Geometry check sheet. Reference: the model listing, model coordinates, mm. A direction names the side the tool comes from. Coordinates: 2 decimals unless noted, no trailing zeros. Loops run counter-clockwise (first coordinate to the right, second up) from the corner with the lowest first, then second, coordinate; pieces in that order, holes last. Notation, with made-up numbers: (30.5, -8.75) - (72.5, -8.75) arc R24 ccw to (72.5, 21.25) - close; hole circle Ø11 at (43, 42.5). An arc over 180 degrees is marked (long way). Write item = value, one per line. Start each with the question number.
Autodesk Inventor part; units mm, degrees
ref_plane "YZ Plane" through (0, 0, 0) normal (1, 0, 0) x (0, 1, 0)
ref_plane "XZ Plane" through (0, 0, 0) normal (0, 1, 0) x (-1, 0, 0)
ref_plane "XY Plane" through (0, 0, 0) normal (0, 0, 1) x (1, 0, 0)
sketch "Sketch1" plane through (0, 0, 0) normal (0, 0, 1) x (1, 0, 0)
  line L0 (0, 0) -> (160, 0)
  line L1 (160, 0) -> (118.589, 154.5481)
  line L2 (41.411, 154.5481) -> (0, 0)
  line L3 (41.411, 154.5481) -> (118.589, 154.5481)
  dimension "d0" = 160
  dimension "d1" = 160
  dimension "d2" = 75
  dimension "d8" = 75
extrude "Extrusion1" add sketch "Sketch1" along normal blind 55
sketch "Sketch6" plane through (0, 0, 55) normal (0, 0, 1) x (1, 0, 0)
  line L0 (0, 0) -> (160, 0) construction
  line L1 (160, 0) -> (118.589, 154.5481) construction
  line L2 (118.589, 154.5481) -> (41.411, 154.5481) construction
  line L3 (41.411, 154.5481) -> (0, 0) construction
  line L4 (110.9157, 144.5481) -> (146.9677, 10) construction
  line L5 (146.9677, 10) -> (13.0323, 10) construction
  line L6 (13.0323, 10) -> (49.0843, 144.5481) construction
  line L7 (49.0843, 144.5481) -> (110.9157, 144.5481) construction
  line L8 (85, 144.5481) -> (75, 144.5481) construction
  line L9 (75, 144.5481) -> (75, 10) construction
  line L10 (75, 10) -> (85, 10) construction
  line L11 (85, 10) -> (85, 144.5481) construction
  line L12 (133.5703, 60) -> (26.4297, 60) construction
  line L13 (26.4297, 60) -> (26.4297, 70) construction
  line L14 (26.4297, 70) -> (133.5703, 70) construction
  line L15 (133.5703, 70) -> (133.5703, 60) construction
  line L16 (133.5703, 60) -> (146.9677, 10)
  line L17 (85, 10) -> (146.9677, 10)
  line L18 (0, 0) -> (160, 0) construction
  line L19 (133.5703, 60) -> (85, 60)
  line L20 (85, 60) -> (85, 10)
  line L21 (75, 10) -> (75, 60)
  line L22 (26.4297, 60) -> (75, 60)
  line L23 (26.4297, 60) -> (13.0323, 10)
  line L24 (13.0323, 10) -> (75, 10)
  line L25 (75, 70) -> (75, 144.5481)
  line L26 (75, 144.5481) -> (49.0843, 144.5481)
  line L27 (75, 70) -> (29.1092, 70)
  line L28 (29.1092, 70) -> (49.0843, 144.5481)
  line L29 (85, 144.5481) -> (110.9157, 144.5481)
  line L30 (110.9157, 144.5481) -> (130.8908, 70)
  line L31 (130.8908, 70) -> (85, 70)
  line L32 (85, 70) -> (85, 144.5481)
  point P0 (80, 10)
  dimension "d22" = 10
  dimension "d23" = 10
  dimension "d24" = 10
  dimension "d25" = 50
extrude "Extrusion5" cut sketch "Sketch6" against normal through all
sketch "Sketch7" plane through (0, 0, 0) normal (0, 0, -1) x (-1, 0, 0)
  circle A0 centre (-80, 304.672) radius 315 construction
  line L0 (0, 0) -> (-160, 0)
  arc A1 (-160, 0) -> (0, 0) centre (-80, 304.672) ccw
  dimension "d28" = 630
extrude "Extrusion6" add sketch "Sketch7" against normal blind 55
sketch "Sketch8" plane through (0, 0, 0) normal (0, 0, -1) x (-1, 0, 0)
  circle A0 centre (-80, 4.836) radius 8.25
  line L0 (-15.7117, 20) -> (-144.2883, 20) construction
  line L1 (-13.0323, 10) -> (-15.7117, 20)
  line L2 (-15.7117, 20) -> (-75, 20)
  line L3 (-75, 10) -> (-75, 60)
  line L4 (-75, 20) -> (-75, 10)
  line L5 (-75, 10) -> (-13.0323, 10)
  line L6 (-75, 10) -> (-13.0323, 10)
  line L7 (-26.4297, 60) -> (-13.0323, 10)
  line L8 (-85, 10) -> (-146.9677, 10)
  line L9 (-146.9677, 10) -> (-144.2883, 20)
  line L10 (-133.5703, 60) -> (-146.9677, 10)
  line L11 (-144.2883, 20) -> (-85, 20)
  line L12 (-85, 60) -> (-85, 10)
  line L13 (-85, 20) -> (-85, 10)
  line L14 (-85, 10) -> (-146.9677, 10)
  line L15 (-118.589, 154.5481) -> (-41.411, 154.5481)
  arc A1 (-160, 0) -> (0, 0) centre (-80, 304.672) ccw
  line L16 (0, -10.328) -> (-160, -10.328) construction
  arc A2 (-160, 0) -> (0, 0) centre (-80, 304.672) ccw
  line L17 (-0.263, 4.836) -> (-159.737, 4.836) construction
  point P0 (-80, 154.5481)
  dimension "d31" = 16.5
  dimension "d32" = 20
extrude "Extrusion8" add sketch "Sketch8" against normal blind 55 contours L5 L3 A0 | A0 L3 L2 L1 L5 | L8 L9 L11 L12 A0 | A0 L12 L8
extrude "Extrusion7" cut sketch "Sketch8" against normal through all contours A0 L8 L12 L3 L5 | L5 L3 A0 | A0 L12 L8
sketch "Sketch9" plane through (15.7117, 20, 0) normal (0, 1, 0) x (1, 0, 0)
  line L0 (0, 0) -> (59.2883, 0)
  line L1 (0, -55) -> (0, 0)
  line L2 (59.2883, -55) -> (0, -55)
  line L3 (59.2883, 0) -> (59.2883, -55)
  line L4 (69.2883, 0) -> (128.5765, 0)
  line L5 (69.2883, -55) -> (69.2883, 0)
  line L6 (128.5765, -55) -> (69.2883, -55)
  line L7 (128.5765, 0) -> (128.5765, -55)
  circle A0 centre (29.6441, -27.5) radius 15
  circle A1 centre (98.9324, -27.5) radius 15
  point P0 (-15.7117, 0)
  point P1 (29.6441, 0)
  point P2 (98.9324, 0)
  point P3 (0, -27.5)
  point P4 (69.2883, -27.5)
  dimension "d37" = 30
  dimension "d38" = 30
extrude "Extrusion9" cut sketch "Sketch9" against normal through all contours A0 | A1
properties part number "CA001" material "ABS Plastic"
(1) Sectioned sample at D-D on x = 53. Enter the section's corners in (y, z), plus the area to 3 significant figures.
(2) Scan lines: line 1 (Y direction, x = 60, z = 5); line 2 (Y direction, x = 90.5, z = 8.5); line 3 (Y direction, x = 54, z = 22). Record each from-to range of solid material in increasing order.
(3) Depth check by flat-ended pin: pin 1 (4 mm diameter, centred on y = 95.5, z = 22.5, fed in from +X); pin 2 (8 mm diameter, centred on x = 65.5, z = 26.5, fed in from -Y); pin 3 (10 mm diameter, centred on y = 101, z = 13.5, fed in from +X). Enter the tip coordinate at first touch or a pass-through.
(4) Sectioned sample at C-C on z = 22.5. Count the separate pieces of the cut face and the enclosed holes in it, plus the area to 3 significant figures.
(5) Tool access check on faces 4 (the face through (75, 107, 28)), 5 (the face through (81, 55, 0)), 6 (the face through (59.21, 5.35, 33.25)). Record the directions out of +Z, -Z, +X, -X, +Y, -Y that give a thin tool (end or side, any length) a straight path to the whole face; none if there is none.
(6) Sectioned sample at A-A on x = 80. Enter the section's corners in (y, z).
(7) Sectioned sample at B-B on y = 122. Enter the section's corners in (x, z).
(8) Draft check along X on faces 1 (the face through (81, 55, 55)), 2 (the face through (62, 144.548, 28)), 3 (the face through (20.995, 78.356, 27.115)). Enter one of: pulls with the +X half, pulls with the -X half, needs draft (parallel to the pull), parting line crosses it, or undercut.
Working result:
q1.outline = (-9.17, 0) - (20, 0) - (20, 14.59) - (-9.17, 14.59) - close; (-9.17, 40.41) - (20, 40.41) - (20, 55) - (-9.17, 55) - close; (60, 0) - (70, 0) - (70, 55) - (60, 55) - close; (144.55, 0) - (154.55, 0) - (154.55, 55) - (144.55, 55) - close
q1.area = 1,950 mm2
q2.line_1 = -9.69 to 20, 60 to 70, 144.55 to 154.55
q2.line_2 = -10.15 to 20, 60 to 70, 144.55 to 154.55
q2.line_3 = 60 to 70, 144.55 to 154.55
q3.pin_1 = 134.95
q3.pin_2 = -10.15
q3.pin_3 = 134.28
q4.separate_pieces = 1
q4.enclosed_holes = 3
q4.area = 7,950 mm2
q5.face_4 = +Z, -Z
q5.face_5 = -Z, +X, -X, +Y, -Y
q5.face_6 = -Y
q6.outline = (-10.33, 0) - (-3.41, 0) - (-3.41, 55) - (-10.33, 55) - close; (13.09, 0) - (154.55, 0) - (154.55, 55) - (13.09, 55) - close
q7.outline = (32.69, 0) - (43.04, 0) - (43.04, 55) - (32.69, 55) - close; (75, 0) - (85, 0) - (85, 55) - (75, 55) - close; (116.96, 0) - (127.31, 0) - (127.31, 55) - (116.96, 55) - close
q8.face_1 = needs draft
q8.face_2 = undercut
q8.face_3 = pulls with the -X half
